Work out the finished part from the listing and answer in its coordinate system (mm). A direction names the side the tool comes from. Coordinates: 2 decimals unless noted, no trailing zeros. Order: outer loops, then holes, each group sorted by start corner. A loop starts at its lowest first (then second) coordinate and runs counter-clockwise, first axis right, second up. Notation, with made-up numbers: M 25,50.5 L 83,50.5 A30 cw 83,89.5 Z; hole C 6,71 d6. An arc over 180 degrees is marked long. Use a Markdown table: item, result. Add a question column.
from build123d import *

# Parameters (mm, degrees)
SKETCH1_W          = 15
SKETCH1_H          = 44
EXTRUDE1_DEPTH     = 40
SKETCH2_W          = 15
SKETCH2_H          = 34
CUT_EXTRUDE1_DEPTH = 32
CUT_EXTRUDE2_DEPTH = 4.3
SKETCH4_R          = 1.25
CUT_EXTRUDE3_DEPTH = 4.3
SKETCH5_R          = 2.5
CUT_EXTRUDE4_DEPTH = 3.3
SKETCH6_W          = 12.4
SKETCH6_H          = 24.4
CUT_EXTRUDE5_DEPTH = 10
SKETCH7_W          = 5
SKETCH7_H          = 3
SKETCH7_W_2        = 2.6
CUT_EXTRUDE6_DEPTH = 12.4
SKETCH8_R          = 1.016
CUT_EXTRUDE7_DEPTH = 20


with BuildPart() as part:
    # Sketch1 → Extrude1 (new body)
    with BuildSketch(Plane.XY):
        with Locations((-19.74138299, 12.778040673)):
            Rectangle(SKETCH1_W, SKETCH1_H)
    extrude(amount=EXTRUDE1_DEPTH)

    # Sketch2 → Cut-Extrude1 (cut)
    with BuildSketch(Plane.XY.offset(40)):
        with Locations((-19.74138299, 12.778040673)):
            Rectangle(SKETCH2_W, SKETCH2_H)
    extrude(amount=-CUT_EXTRUDE1_DEPTH, mode=Mode.SUBTRACT)

    # Sketch3 → Cut-Extrude2 (cut)
    with BuildSketch(Plane(origin=(0, 0, 0), x_dir=(-1, 0, 0), z_dir=(0, 0, -1))):
        Polygon((22.49138299, 10.028040673), (27.24138299, 10.028040673), (27.24138299, 15.528040673), (22.49138299, 15.528040673), (22.49138299, 27.528040673), (16.99138299, 27.528040673), (16.99138299, 15.528040673), (12.24138299, 15.528040673), (12.24138299, 10.028040673), (16.99138299, 10.028040673), (16.99138299, -1.971959327), (22.49138299, -1.971959327), align=None)
    extrude(amount=-CUT_EXTRUDE2_DEPTH, mode=Mode.SUBTRACT)

    # Sketch4 → Cut-Extrude3 (cut)
    with BuildSketch(Plane(origin=(0, 0, 4.3), x_dir=(-1, 0, 0), z_dir=(0, 0, -1))):
        with Locations((19.74138299, 12.778040673)):
            Circle(SKETCH4_R)
    extrude(amount=-CUT_EXTRUDE3_DEPTH, mode=Mode.SUBTRACT)

    # Sketch5 → Cut-Extrude4 (cut)
    with BuildSketch(Plane.XY.offset(8)):
        with Locations((-19.74138299, 12.778040673)):
            Circle(SKETCH5_R)
    extrude(amount=-CUT_EXTRUDE4_DEPTH, mode=Mode.SUBTRACT)

    # Sketch6 → Cut-Extrude5 (cut)
    with BuildSketch(Plane(origin=(0, -4.221959327, 0), x_dir=(1, 0, 0), z_dir=(0, 1, 0))):
        with Locations((-18.44138299, -22.8)):
            Rectangle(SKETCH6_W, SKETCH6_H)
    cut_extrude5 = extrude(amount=-CUT_EXTRUDE5_DEPTH, mode=Mode.SUBTRACT)

    # Sketch7 → Cut-Extrude6 (cut)
    with BuildSketch(Plane(origin=(-12.24138299, 0, 0), x_dir=(0, 0, -1), z_dir=(1, 0, 0))):
        with Locations((-37.5, -5.721959327)):
            Rectangle(SKETCH7_W, SKETCH7_H)
        with Locations((-9.3, -5.721959327)):
            Rectangle(SKETCH7_W_2, SKETCH7_H)
    cut_extrude6 = extrude(amount=-CUT_EXTRUDE6_DEPTH, mode=Mode.SUBTRACT)

    # Sketch8 → Cut-Extrude7 (cut)
    with BuildSketch(Plane.XZ.offset(9.221959327)):
        with Locations((-21.90518052, 36.578)):
            Circle(SKETCH8_R)
        with Locations(Location((-14.977585459, 36.578, 0), (0, 0, 270))):
            Circle(SKETCH8_R)
        with Locations((-14.977585459, 9.022)):
            Circle(SKETCH8_R)
        with Locations(Location((-21.90518052, 9.022, 0), (0, 0, 270))):
            Circle(SKETCH8_R)
    cut_extrude7 = extrude(amount=-CUT_EXTRUDE7_DEPTH, mode=Mode.SUBTRACT)

    # Mirror1: Cut-Extrude5, Cut-Extrude6, Cut-Extrude7 across plane
    add(cut_extrude5.mirror(Plane(origin=(0, 12.778040673, 0), x_dir=(0, 0, 1), z_dir=(0, -1, 0))), mode=Mode.SUBTRACT)
    add(cut_extrude6.mirror(Plane(origin=(0, 12.778040673, 0), x_dir=(0, 0, 1), z_dir=(0, -1, 0))), mode=Mode.SUBTRACT)
    add(cut_extrude7.mirror(Plane(origin=(0, 12.778040673, 0), x_dir=(0, 0, 1), z_dir=(0, -1, 0))), mode=Mode.SUBTRACT)


solid = part.part
(1) A cutting plane is placed at B-B on z = 15. Write down the section's boundary in (x, y).
(2) A cutting plane is placed at A-A on x = -24. Write down the section's boundary in (y, z), plus the area to 3 significant figures.
(3) A cutting plane is placed at D-D on y = -2.5. Write down the section's boundary in (x, z).
(4) Which of the six approach directions +Z, -Z, +X, -X, +Y, -Y give full straight-line access (tool end or side, diameter ignored) to faces 4 (the flat face through (-15, 15.528, 2)), 5 (the flat face through (-19, -8, 35)), 6 (the cylindrical face through (-17.357, 13.529, 6.373)), 7 (the flat face through (-18, 32.778, 38)), 8 (the flat face through (-20, 27.528, 2))?
(5) Given P1, Ø1, axis at x = -21, y = 3.5, coming from the -Z side; P2, Ø2.5, axis at y = -6, z = 31, coming from the +X side; P3, Ø4.5, axis at x = -19.74, y = 12.78, coming from the +Z side, each flat-ended and moving along its own axis, determine where each tip first touches the part or whether it passes through.
(6) A cutting plane is placed at C-C on y = 20. Write down the section's boundary in (x, z).
(7) Straight lines are drawn through the part: line 1 (Y direction, x = -25.5, z = 23); line 2 (Y direction, x = -20, z = 4); line 3 (X direction, y = 30.5, z = 30). For each, find the intervals that lie inside material, in ascending order.
(8) The mould has two halves that part along X. Classify faces 1 (the flat face through (-20, -4, 0)), 2 (the flat face through (-24.641, -7, 24)), 3 (the cylindrical face through (-21.6, 33.792, 8.053)): pulls with the +X half, pulls with the -X half, needs draft (parallel to the pull), parting line crosses it, or undercut.
From the geometry:
| question | item | result |
|---|---|---|
| 1 | outline | M -27.24,-9.22 L -24.64,-9.22 L -24.64,-4.22 L -27.24,-4.22 Z; M -27.24,29.78 L -24.64,29.78 L -24.64,34.78 L -27.24,34.78 Z |
| 2 | outline | M -9.22,0 L 10.03,0 L 10.03,4.3 L 15.53,4.3 L 15.53,0 L 34.78,0 L 34.78,10.6 L 32.78,10.6 L 32.78,8 L -7.22,8 L -7.22,10.6 L -9.22,10.6 Z; M -9.22,35 L -7.22,35 L -7.22,40 L -9.22,40 Z; M 32.78,35 L 34.78,35 L 34.78,40 L 32.78,40 Z |
| 2 | area | 359 mm2 |
| 3 | outline | M -27.24,0 L -12.24,0 L -12.24,8 L -27.24,8 Z |
| 4 | face 4 | -Z, +X, -X |
| 4 | face 5 | +X, +Y, -Y |
| 4 | face 6 | +Z |
| 4 | face 7 | +Z, +X |
| 4 | face 8 | -Z |
| 5 | P1 | stops at z = 4.3 |
| 5 | P2 | stops at x = -24.64 |
| 5 | P3 | stops at z = 4.7 |
| 6 | outline | M -27.24,0 L -22.49,0 L -22.49,4.3 L -16.99,4.3 L -16.99,0 L -12.24,0 L -12.24,8 L -27.24,8 Z |
| 7 | line 1 | y = -9.22 to -4.22, 29.78 to 34.78 |
| 7 | line 2 | y = -9.22 to -1.97, 27.53 to 34.78 |
| 7 | line 3 | x = -27.24 to -24.64 |
| 8 | face 1 | needs draft |
| 8 | face 2 | pulls with the +X half |
| 8 | face 3 | undercut |
